from build123d import *

# Parameters (mm, degrees)
BOSS_EXTRUDE1_DEPTH = 36
CUT_EXTRUDE1_REACH  = 21.399
CUT_EXTRUDE2_REACH  = 21.399
BOSS_EXTRUDE2_DEPTH = 2
CUT_EXTRUDE3_REACH  = 11
SKETCH5_W           = 5
SKETCH5_H           = 17
CUT_EXTRUDE4_REACH  = 21.399
SKETCH6_R           = 1.5


with BuildPart() as part:
    # Sketch1 → Boss-Extrude1 (new body)
    with BuildSketch(Plane(origin=(0, 0, 0), x_dir=(1, 0, 0), z_dir=(0, 1, 0))):
        Polygon((0, 0), (11.909668113, 0), (14.399319728, 2.489651615), (17.399319728, 2.489651615), (17.399319728, 21), (19.399319728, 21), (19.399319728, 1.06122449), (15.799319728, 1.06122449), (12.738095238, -2), (10, -2), (10, -9), (0, -9), align=None)
    extrude(amount=BOSS_EXTRUDE1_DEPTH)

    # Sketch2 → Cut-Extrude1 (cut, up to next)
    with BuildSketch(Plane(origin=(19.399319728, 0, 0), x_dir=(0, 0, -1), z_dir=(1, 0, 0)), mode=Mode.PRIVATE) as cut_extrude1_sk1:
        Polygon((3.06122449, 36), (3.06122449, 33), (21, 7.380773512), (21, 36), align=None)
    cut_extrude1_tool1 = extrude(cut_extrude1_sk1.sketch, amount=-CUT_EXTRUDE1_REACH, mode=Mode.PRIVATE) & part.part
    add(cut_extrude1_tool1.solids().sort_by_distance((19.39932, 26.365379, -14.453071))[0], mode=Mode.SUBTRACT)

    # Sketch3 → Cut-Extrude2 (cut, up to next)
    with BuildSketch(Plane(origin=(19.399319728, 0, 0), x_dir=(0, 0, -1), z_dir=(1, 0, 0)), mode=Mode.PRIVATE) as cut_extrude2_sk1:
        with BuildLine():
            Line((6.80922077, 19.075125289), (13.914682933, 9.520466295))
            ThreePointArc((13.914682933, 9.520466295), (14.061573755, 9.238022803), (14.112249375, 8.923724822))
            Line((14.112249375, 8.923724822), (14.112249375, 6.370604423))
            ThreePointArc((14.112249375, 6.370604423), (13.819356156, 5.663497642), (13.112249375, 5.370604423))
            Line((13.112249375, 5.370604423), (6.006787212, 5.370604423))
            ThreePointArc((6.006787212, 5.370604423), (5.299680431, 5.663497642), (5.006787212, 6.370604423))
            Line((5.006787212, 6.370604423), (5.006787212, 18.478383816))
            ThreePointArc((5.006787212, 18.478383816), (5.692489231, 19.427708197), (6.80922077, 19.075125289))
        make_face()
    cut_extrude2_tool1 = extrude(cut_extrude2_sk1.sketch, amount=-CUT_EXTRUDE2_REACH, mode=Mode.PRIVATE) & part.part
    add(cut_extrude2_tool1.solids().sort_by_distance((19.39932, 10.844583, -8.68829))[0], mode=Mode.SUBTRACT)

    # Sketch4 → Boss-Extrude2 (add)
    with BuildSketch(Plane(origin=(19.399319728, 0, 0), x_dir=(0, 0, -1), z_dir=(1, 0, 0))):
        with BuildLine():
            Line((21, 0), (21, -3))
            ThreePointArc((21, -3), (17, -7), (13, -3))
            Line((13, -3), (13, 0))
            Line((13, 0), (21, 0))
        make_face()
    extrude(amount=-BOSS_EXTRUDE2_DEPTH)

    # Sketch5 → Cut-Extrude3 (cut, up to next)
    with BuildSketch(Plane(origin=(0, 0, 0), x_dir=(-1, 0, 0), z_dir=(0, 0, -1)), mode=Mode.PRIVATE) as cut_extrude3_sk1:
        with Locations((-2.5, 19.5)):
            Rectangle(SKETCH5_W, SKETCH5_H)
    cut_extrude3_tool1 = extrude(cut_extrude3_sk1.sketch, amount=-CUT_EXTRUDE3_REACH, mode=Mode.PRIVATE) & part.part
    add(cut_extrude3_tool1.solids().sort_by_distance((2.5, 19.5, 0))[0], mode=Mode.SUBTRACT)

    # Sketch6 → Cut-Extrude4 (cut, up to next)
    with BuildSketch(Plane(origin=(19.399319728, 0, 0), x_dir=(0, 0, -1), z_dir=(1, 0, 0)), mode=Mode.PRIVATE) as cut_extrude4_sk1:
        with Locations((17, -1)):
            Circle(SKETCH6_R)
    cut_extrude4_tool1 = extrude(cut_extrude4_sk1.sketch, amount=-CUT_EXTRUDE4_REACH, mode=Mode.PRIVATE) & part.part
    add(cut_extrude4_tool1.solids().sort_by_distance((19.39932, -1, -17))[0], mode=Mode.SUBTRACT)


solid = part.part
For this review, take the finished solid that the model builds, in its own axes (mm). A direction names the side the tool comes from. Round coordinates to 2 decimals unless told otherwise and drop trailing zeros. Loops run counter-clockwise (first coordinate to the right, second up) from the corner with the lowest first, then second, coordinate; pieces in that order, holes last. Notation, with made-up numbers: (-18, 29.5) - (-5, 29.5) arc R22 cw to (-5, 68.5) - close; hole circle Ø11 at (-15.5, 35.5). An arc over 180 degrees is marked (long way). One line per question, with ' | ' between items.
Q1. The part is to be moulded in two halves that separate along Y. For faces 1 (the flat face through (18.413, 20.37, -11.905)), 2 (the flat face through (18, 35, -3.061)), 3 (the cylindrical face through (18.413, 19.422, -5.676)), 4 (the cylindrical face through (18, -7, -17)), say which applies: released by +Y, released by -Y, zero draft, split by the parting line, or undercut.
Taken from the geometry:
face 1: released by +Y | face 2: zero draft | face 3: undercut | face 4: released by -Y
Q2. Tool access review of faces 5 (the flat face through (17.399, 10, -14)), 6 (the flat face through (18, -2, -13)), 7 (the flat face through (18.413, 14.365, -10.312)), 8 (the flat face through (3, 11, 4)): name each direction out of +Z, -Z, +X, -X, +Y, -Y from which nothing blocks a thin tool from reaching the whole face with its end or side.
Taken from the geometry:
face 5: -Z, -X, +Y, -Y | face 6: +Z, +X, -X, -Y | face 7: +X, -X | face 8: +Z, -Z, -X
Q3. Take a section at A-A (x = 1.5). Give the boundary of the cut face in (y, z), and give its area (3 significant figures).
Taken from the geometry:
outline: (0, 0) - (11, 0) - (11, 9) - (0, 9) - close; (28, 0) - (36, 0) - (36, 9) - (28, 9) - close | area: 171 mm²
Q4. Take a section at D-D (y = 23.5). Give the boundary of the cut face in (x, z), and give its area (3 significant figures).
Taken from the geometry:
outline: (5, 0) - (11.91, 0) - (14.4, -2.49) - (17.4, -2.49) - (17.4, -9.71) - (19.4, -9.71) - (19.4, -1.06) - (15.8, -1.06) - (12.74, 2) - (10, 2) - (10, 9) - (5, 9) - close | area: 78.1 mm²
Q5. Take a section at C-C (y = 12.5). Give the boundary of the cut face in (x, z), and give its area (3 significant figures).
Taken from the geometry:
outline: (5, 0) - (11.91, 0) - (14.4, -2.49) - (17.4, -2.49) - (17.4, -5.01) - (19.4, -5.01) - (19.4, -1.06) - (15.8, -1.06) - (12.74, 2) - (10, 2) - (10, 9) - (5, 9) - close; (17.4, -17.42) - (19.4, -17.42) - (19.4, -11.7) - (17.4, -11.7) - close | area: 80.1 mm²
Q6. Take a section at B-B (y = -1). Give the boundary of the cut face in (x, z).
Taken from the geometry:
outline: (17.4, -21) - (19.4, -21) - (19.4, -18.5) - (17.4, -18.5) - close; (17.4, -15.5) - (19.4, -15.5) - (19.4, -13) - (17.4, -13) - close
Q7. For line 1 along Z through (x, y) = (16, 31.5); line 2 along Y through (x, z) = (18.25, -1.5); line 3 along Z through (x, y) = (18, 6.5), list the stretches that pass through material, from the lowest coordinate up. Write a range as [from, to].
Taken from the geometry:
line 1: z = [-2.49, -1.06] | line 2: y = [0, 36] | line 3: z = [-21, -14.11], [-5.01, -1.06]
Q8. For pin 1 (1.8 mm diameter, centred on x = 17, y = 19, fed in from +Z); pin 2 (1.5 mm diameter, centred on x = 14.5, y = 23, fed in from -Z); pin 3 (1.6 mm diameter, centred on x = 18.5, y = -1.5, fed in from +Z), all flat-tipped, find the tip position at first contact; note any pin that passes through.
Taken from the geometry:
pin 1: stops at z = -1.06 | pin 2: stops at z = -2.49 | pin 3: stops at z = -13
